Source: CAD feature listing. Evaluate the final solid. Frame: model axes, mm. Give positions to 0.01 mm unless a question says otherwise; leave off trailing zeros. Write each loop counter-clockwise with the first axis right and the second up, starting at its lowest first coordinate (ties: lowest second). Pieces come first, ordered by that corner, then holes. Notation, with made-up numbers: (-19, -23.5) -> (7, -23.5) arc R26 cw to (7, -3.5) -> close; hole circle Ø10 at (47.5, 15.5). An arc over 180 degrees is marked (long way). Write item = value, one per line.
from build123d import *

# Parameters (mm, degrees)
SKETCH2_W           = 63
SKETCH2_H           = 53.66
SKETCH2_R           = 5.25
SKETCH2_R_2         = 11.25
BOSS_EXTRUDE1_DEPTH = 15
SKETCH3_R           = 5.35
CUT_EXTRUDE1_DEPTH  = 71.244392635


with BuildPart() as part:
    # Sketch2 → Boss-Extrude1 (new body)
    with BuildSketch(Plane.XY):
        with Locations((-0.443782019, -0.377989574)):
            Rectangle(SKETCH2_W, SKETCH2_H)
        with Locations((23.056217981, 13.452010426)):
            Circle(SKETCH2_R, mode=Mode.SUBTRACT)
        with Locations((-16.943782019, 13.452010426)):
            Circle(SKETCH2_R_2, mode=Mode.SUBTRACT)
    extrude(amount=BOSS_EXTRUDE1_DEPTH)

    # Sketch3 → Cut-Extrude1 (cut, through all)
    with BuildSketch(Plane(origin=(31.056217981, 0, 0), x_dir=(0, 0, -1), z_dir=(1, 0, 0))):
        with Locations((-7.5, -20.207989574)):
            Circle(SKETCH3_R)
    extrude(amount=-CUT_EXTRUDE1_DEPTH, mode=Mode.SUBTRACT)


solid = part.part
(1) Section query D-D (x = 15.5). Return loops of the section in (y, z), plus the area to 3 significant figures.
Values follow:
outline = (-27.21, 0) -> (26.45, 0) -> (26.45, 15) -> (-27.21, 15) -> close; hole circle Ø10.7 at (-20.21, 7.5)
area = 715 mm2
(2) Material intervals for line 1 (Y direction, x = -12, z = 6); line 2 (Y direction, x = -7, z = 11); line 3 (X direction, y = 14.5, z = 12.75), sorted ascending.
Values follow:
line_1 = -27.21 to -25.34, -15.07 to 3.35, 23.56 to 26.45
line_2 = -27.21 to -24.25, -16.16 to 8.19, 18.71 to 26.45
line_3 = -31.94 to -28.14, -5.74 to 17.91, 28.2 to 31.06
(3) Section query B-B (x = -25). Return loops of the section in (y, z).
Values follow:
outline = (-27.21, 0) -> (5.6, 0) -> (5.6, 15) -> (-27.21, 15) -> close; (21.3, 0) -> (26.45, 0) -> (26.45, 15) -> (21.3, 15) -> close; hole circle Ø10.7 at (-20.21, 7.5)
(4) First-contact query: pin 1 (8.5 mm diameter, centred on y = -20.21, z = 7.5, fed in from -X). Flat tip, straight axial feed; report the tip coordinate or a pass-through.
Values follow:
pin_1 = through
(5) Section query A-A (z = 6). Return loops of the section in (x, y).
Values follow:
outline = (-31.94, -27.21) -> (31.06, -27.21) -> (31.06, -25.34) -> (-31.94, -25.34) -> close; (-31.94, -15.07) -> (31.06, -15.07) -> (31.06, 26.45) -> (-31.94, 26.45) -> close; hole circle Ø22.5 at (-16.94, 13.45); hole circle Ø10.5 at (23.06, 13.45)
(6) Section query C-C (y = 6). Return loops of the section in (x, z).
Values follow:
outline = (-31.94, 0) -> (-25.37, 0) -> (-25.37, 15) -> (-31.94, 15) -> close; (-8.52, 0) -> (31.06, 0) -> (31.06, 15) -> (-8.52, 15) -> close
(7) Pull-direction query (Y, two-part tool) for faces 1 (the face through (-6.552, 9.143, 7.395)), 2 (the face through (-1, -27.208, 7)), 3 (the face through (-1, 0, 15)); classes: pulls with the +Y half, pulls with the -Y half, needs draft (parallel to the pull), parting line crosses it, or undercut.
Values follow:
face_1 = undercut
face_2 = pulls with the -Y half
face_3 = needs draft
